from build123d import *

# Parameters (mm, degrees)
F1_DEPTH = 63.5
F0_W     = 10.8645128564
F0_H     = 19.05
F2_DEPTH = 25.4
F3_DEPTH = 7.9375
F5_R     = 6.35


with BuildPart() as f1:
    # F0 (on Front) → F1 (new body, symmetric)
    with BuildSketch(Plane.XZ):
        Polygon((-41.275, -9.525), (41.275, -9.525), (41.275, 9.525), (22.225, 9.525), (-41.275, 9.525), align=None)
    extrude(amount=F1_DEPTH, both=True)

    # F0 (on Front) → F2 (join, symmetric)
    with BuildSketch(Plane.XZ):
        with BuildLine():
            Line((22.225, 9.525), (41.275, 9.525))
            Line((41.275, 9.525), (41.275, 28.8110316193))
            ThreePointArc((41.275, 28.8110316193), (43.5686828026, 37.0307304084), (49.7869304797, 42.8752))
            Line((49.7869304797, 42.8752), (60.325, 42.8752))
            Line((60.325, 42.8752), (60.325, 61.9252))
            Line((60.325, 61.9252), (46.0501136286, 61.9252))
            ThreePointArc((46.0501136286, 61.9252), (28.8002278976, 49.2082384561), (22.225, 28.8110316193))
            Line((22.225, 28.8110316193), (22.225, 9.525))
        make_face()
        with Locations((65.7572564282, 52.4002)):
            Rectangle(F0_W, F0_H)
    extrude(amount=F2_DEPTH, both=True)

    # F0 (on Front) → F3 (join, symmetric)
    with BuildSketch(Plane.XZ):
        with BuildLine():
            add(Edge.make_bspline(
                [(-41.275, 9.525), (-40.2269773185, 37.5649705529), (16.0009935498, 65.2335137129), (46.0501136286, 61.9252)],
                knots=[0, 0, 0, 0, 101.8403477522, 101.8403477522, 101.8403477522, 101.8403477522], degree=3))
            Line((-41.275, 9.525), (22.225, 9.525))
            Line((22.225, 9.525), (22.225, 28.8110316193))
            ThreePointArc((22.225, 28.8110316193), (28.8002278976, 49.2082384561), (46.0501136286, 61.9252))
        make_face()
    extrude(amount=F3_DEPTH, both=True)

    # F0 (on Front) → F4 (revolve)
    with BuildSketch(Plane.XZ):
        Polygon((60.325, 66.675), (60.325, 61.9252), (71.1895128564, 61.9252), (71.1895128564, 42.8752), (60.325, 42.8752), (60.325, 38.1), (111.125, 38.1), (111.125, 66.675), align=None)
    revolve(axis=Axis((60.325, 0, 52.3875), (0, 0, 1)))

    # F5
    f5_edges = [f1.edges().sort_by_distance(p)[0] for p in [
        (-41.275, -63.5, 0),
        (41.275, -63.5, 0),
        (41.275, 63.5, 0),
        (-41.275, 63.5, 0),
    ]]
    fillet(f5_edges, radius=F5_R)


solid = f1.part
The listing builds one solid part. Answer for the finished solid, in the listing's coordinates (mm). A direction names the side the tool comes from. Round coordinates to 2 decimals unless told otherwise and drop trailing zeros. Write each loop counter-clockwise with the first axis right and the second up, starting at its lowest first coordinate (ties: lowest second). Pieces come first, ordered by that corner, then holes. Notation, with made-up numbers: (59, 28.25) - (109, 28.25) arc R20 ccw to (109, 60.25) - close; hole circle Ø11 at (82, 38.5). An arc over 180 degrees is marked (long way). Use a Markdown table: item, result. Add a question column.
1. The part is cut by section B-B (z = 4). Write down the section's boundary in (x, y) (3 decimals).
2. A tool of negligible diameter and unlimited length cuts with its end or side. For faces 1 (the face through (39.464, 61.59, 0.133)), 2 (the face through (60, 1, 66.675)), 3 (the face through (33, 25.4, 24)), 4 (the face through (-8, -7.938, 28)), 5 (the face through (22.225, 17, 19)), from which of +Z, -Z, +X, -X, +Y, -Y can it reach the whole face along a straight path? Write none if from no direction.
3. Flat-ended cylindrical pins translate along their axes: P1, Ø12, axis at x = 10, z = 31, coming from the +Y side; P2, Ø6.5, axis at x = 32, z = 22.5, coming from the -Y side; P3, Ø3, axis at y = -21, z = 7.5, coming from the +X side (3 decimals). Find the tip coordinate at first contact, or state that the pin passes through.
4. For a pull along Z with two mould halves and no side action, classify faces 6 (the face through (42.023, -0.356, 33.626)), 7 (the face through (-39.464, 61.59, -0.133)), 8 (the face through (33, -25.4, 24)) as +Z half, -Z half, draft (parallel to the pull), parting line (faces both ways), or undercut.
5. The part is cut by section D-D (y = -21). Write down the section's boundary in (x, z) (3 decimals), and give its area (3 significant figures).
6. The part is cut by section C-C (x = 38.5). Write down the section's boundary in (y, z) (3 decimals).
7. The part is cut by section A-A (y = -40). Write down the section's boundary in (x, z) (3 decimals).
8. Consider line 1 (Z direction, x = 17.5, y = 25) (3 decimals); line 2 (Z direction, x = 22, y = 49.5) (3 decimals); line 3 (Z direction, x = 96, y = 18) (3 decimals). Determine where each line is inside the solid, lowest interval first.
Reported:
| question | item | result |
|---|---|---|
| 1 | outline | (-41.275, -57.15) arc R6.35 ccw to (-34.925, -63.5) - (34.925, -63.5) arc R6.35 ccw to (41.275, -57.15) - (41.275, 57.15) arc R6.35 ccw to (34.925, 63.5) - (-34.925, 63.5) arc R6.35 ccw to (-41.275, 57.15) - close |
| 2 | face 1 | +Z, -Z, +X, +Y |
| 2 | face 2 | +Z, +X, -X, +Y, -Y |
| 2 | face 3 | +X, -X, +Y |
| 2 | face 4 | -X, -Y |
| 2 | face 5 | -X, +Y |
| 3 | P1 | y = 7.94 |
| 3 | P2 | y = -25.4 |
| 3 | P3 | x = 41.275 |
| 4 | face 6 | -Z half |
| 4 | face 7 | draft |
| 4 | face 8 | undercut |
| 5 | outline | (-41.275, -9.525) - (41.275, -9.525) - (41.275, 28.811) arc R15.875 cw to (44.276, 38.1) - (106.581, 38.1) - (106.581, 66.675) - (14.069, 66.675) - (14.069, 38.1) - (23.483, 38.1) arc R34.925 ccw to (22.225, 28.811) - (22.225, 9.525) - (-41.275, 9.525) - close |
| 5 | area | 4,770 mm^2 |
| 6 | outline | (-62.398, -9.525) - (62.398, -9.525) - (62.398, 9.525) - (25.4, 9.525) - (25.4, 38.1) - (45.873, 38.1) - (45.873, 66.675) - (-45.873, 66.675) - (-45.873, 38.1) - (-25.4, 38.1) - (-25.4, 9.525) - (-62.398, 9.525) - close |
| 7 | outline | (-41.275, -9.525) - (41.275, -9.525) - (41.275, 9.525) - (-41.275, 9.525) - close; (29.01, 38.1) - (91.64, 38.1) - (91.64, 66.675) - (29.01, 66.675) - close |
| 8 | line 1 | -9.525 to 9.525, 38.1 to 66.675 |
| 8 | line 2 | -9.525 to 9.525 |
| 8 | line 3 | 38.1 to 66.675 |
